Work out the finished part from the listing and answer in its coordinate system (mm). A direction names the side the tool comes from. Coordinates: 2 decimals unless noted, no trailing zeros. Write each loop counter-clockwise with the first axis right and the second up, starting at its lowest first coordinate (ties: lowest second). Pieces come first, ordered by that corner, then holes. Notation, with made-up numbers: (10.5, -23) -> (46.5, -23) arc R14 ccw to (46.5, 4) -> close; hole circle Ø1 at (87, 87.25). An arc over 180 degrees is marked (long way). Write each question's results on one line, items separated by ' | '. Start each with the question number.
Autodesk Inventor part; units mm, degrees
ref_plane "YZ Plane" through (0, 0, 0) normal (1, 0, 0) x (0, 1, 0)
ref_plane "XZ Plane" through (0, 0, 0) normal (0, 1, 0) x (-1, 0, 0)
ref_plane "XY Plane" through (0, 0, 0) normal (0, 0, 1) x (1, 0, 0)
sketch "Skizze1" plane through (0, 0, 0) normal (0, 0, 1) x (1, 0, 0)
  circle A0 centre (3.625, -20.7) radius 1.6
  circle A1 centre (3.625, -7) radius 1.6
  line L0 (7.8, -27.7) -> (7.8, -25.75)
  line L1 (7.8, -25.75) -> (7.25, -25.75)
  line L2 (7.25, -25.75) -> (7.25, 0)
  line L3 (0, 0) -> (7.25, 0)
  line L4 (0, -27.7) -> (0, 0)
  line L5 (0, -27.7) -> (7.8, -27.7)
  circle A2 centre (13.375, -20.7) radius 1.6
  circle A3 centre (13.375, -7) radius 1.6
  line L6 (9.2, -25.75) -> (9.2, -27.7)
  line L7 (9.2, -27.7) -> (17, -27.7)
  line L8 (17, 0) -> (17, -27.7)
  line L9 (9.75, 0) -> (17, 0)
  line L10 (9.75, 0) -> (9.75, -25.75)
  line L11 (9.75, -25.75) -> (9.2, -25.75)
  line L12 (0.5, 0) -> (17, 0)
  line L13 (17, 0) -> (17, -27.7)
  line L14 (17, -27.7) -> (0.5, -27.7)
  line L15 (0.5, -27.7) -> (0.5, 0)
  dimension "d0" = 0.5
extrude "Extrusion1" add sketch "Skizze1" along normal blind 5 contours A0 | A1 | L5 L15 L3 L2 L1 L0 | L0 L1 L2 L12 L10 L11 L6 L14 | L6 L11 L10 L9 L8 L7 | A2 | A3
sketch "Skizze2" plane through (0, 0, 5) normal (0, 0, 1) x (1, 0, 0)
  circle A0 centre (3.625, -7) radius 1.6
  circle A1 centre (13.375, -7) radius 1.6
  circle A2 centre (13.375, -20.7) radius 1.6
  circle A3 centre (3.625, -20.7) radius 1.6
  point P0 (0, 0)
extrude "Extrusion2" cut sketch "Skizze2" against normal blind 10
sketch "Skizze3" plane through (0, 0, 0) normal (0, 0, -1) x (-1, 0, 0)
  line L0 (-7.25, -25.75) -> (-7.25, 0)
  line L1 (-9.75, 0) -> (-9.75, -25.75)
  line L2 (-9.75, -25.75) -> (-7.25, -25.75)
  line L3 (-7.25, 0) -> (-9.75, 0)
  line L4 (-17, 0) -> (-0.5, 0)
  point P0 (0, 0)
  dimension "d5" = 2.5
extrude "Extrusion3" cut sketch "Skizze3" against normal blind 1.25
sketch "Skizze4" plane through (0, 0, 0) normal (0, 0, -1) x (-1, 0, 0)
  line L0 (-7.8, -27.7) -> (-7.8, -25.75)
  line L1 (-9.2, -25.75) -> (-9.2, -27.7)
  line L2 (-7.8, -27.7) -> (-9.2, -27.7)
  line L3 (-0.5, -27.7) -> (-17, -27.7)
  line L4 (-7.8, -25.75) -> (-9.2, -25.75)
  line L5 (-7.25, -25.75) -> (-9.75, -25.75)
  point P0 (0, 0)
  dimension "d8" = 1.4
extrude "Extrusion4" cut sketch "Skizze4" against normal blind 0.7
fillet "Rundung1" radius 2 2 edges at (17, 0, 2.5) (17, -27.7, 2.5)
sketch "Skizze5" plane through (0.5, 0, 5) normal (0, 1, 0) x (1, 0, 0)
  line L0 (0, 5) -> (7.3, 5)
  line L1 (8.7, 5) -> (14.5, 5)
  arc A0 (5.5, 5) -> (10.5, 5) centre (8, 5) ccw
  line L2 (8.7, 4.3) -> (7.3, 4.3)
  arc A1 (3, 5) -> (13, 5) centre (8, 5) ccw
  line L3 (13, 5) -> (10.5, 5)
  line L4 (5.5, 5) -> (3, 5)
  line L5 (14.5, 0) -> (0, 0)
  point P0 (-0.5, 5)
  point P1 (8, 4.3)
  dimension "d12" = 2.5
  dimension "d13" = 0
extrude "Extrusion5" add sketch "Skizze5" along normal blind 20
sketch "Skizze7" plane through (0, 0, 5) normal (0, 0, 1) x (1, 0, 0)
  circle A0 centre (3.625, -7) radius 3
  circle A1 centre (13.375, -7) radius 3
  circle A2 centre (13.375, -20.7) radius 1.6
  circle A3 centre (13.375, -20.7) radius 3
  circle A4 centre (3.625, -20.7) radius 3
  circle A5 centre (3.625, -7) radius 1.6
  circle A6 centre (13.375, -7) radius 1.6
  circle A7 centre (3.625, -20.7) radius 1.6
  point P0 (0, 0)
  dimension "d18" = 6
extrude "Extrusion7" cut sketch "Skizze7" against normal blind 2 contours A0 | A1 | A2 | A3 | A4 | A5 | A7
sketch "Skizze8" plane through (0.5, 20, 5) normal (0, 1, 0) x (1, 0, 0)
  point P0 (-0.5, 5)
sketch "Skizze9" plane through (0.5, 20, 5) normal (0, 1, 0) x (1, 0, 0)
  line L0 (13, 5) -> (10.5, 5)
  arc A0 (5.5, 5) -> (10.5, 5) centre (8, 5) ccw
  line L1 (5.5, 5) -> (3, 5)
  arc A1 (3, 5) -> (13, 5) centre (8, 5) ccw
  circle A2 centre (8, 5) radius 5
  line L2 (5.5, 5) -> (10.5, 5)
  point P0 (-0.5, 5)
  point P1 (3, 5)
  point P2 (13, 5)
extrude "Extrusion8" add sketch "Skizze9" along normal blind 2 contours A1 L1 A0 L0 | A0 L2
equation "\"d6\" = 0.5 * d5"
equation "\"d9\" = 0.5 * d8"
properties part number "NadelHalterLose"
1. Given pin 1 Ø1 at (x, z) = (2.5, 3.5) entering from +Y; pin 2 Ø5 at (x, y) = (3.625, -20.7) entering from -Z; pin 3 Ø1.5 at (x, y) = (4.5, -20.5) entering from +Z; pin 4 Ø0.7 at (x, y) = (8.5, -26.5) entering from -Z, each flat-ended and moving along its own axis, determine where each tip first touches the part or whether it passes through.
2. Find the intervals of material crossed by L1, parallel to Y at x = 3.5, z = 3.55; L2, parallel to Y at x = 4, z = 2.85; L3, parallel to Y at x = 8.75, z = 1.8, in increasing order.
3. Find section D-D on y = 16. Give the vertices of the cut face in (x, z), and give its area (3 significant figures).
4. Determine the mould class of faces 1 (the face through (8, 20, 1)), 2 (the face through (0.5, -14, 2)), 3 (the face through (16.43, -0.6, 2.54)), 4 (the face through (8, 0, 2)) for opening direction Y: pulls with the +Y half, pulls with the -Y half, needs draft (parallel to the pull), parting line crosses it, or undercut.
5. Find section C-C on y = -16. Give the vertices of the cut face in (x, z), and give its area (3 significant figures).
6. Find section B-B on z = 3.6. Give the vertices of the cut face in (x, y) (3 decimals), and give its area (3 significant figures).
7. For faces 5 (the face through (7.25, -13, 1)), 6 (the face through (8, 22, 2)), 7 (the face through (1.414, -4.972, 4.014)), 8 (the face through (3, 0, 3)), determine the directions among +Z, -Z, +X, -X, +Y, -Y from which every point of the face is accessible in a straight line to the end or side of a thin tool.
8. Find section A-A on y = -7. Give the vertices of the cut face in (x, z) (3 decimals), and give its area (3 significant figures).
Ans:
1) pin 1: stops at y = 0 | pin 2: stops at z = 0 | pin 3: stops at z = 3 | pin 4: stops at z = 0.7
2) L1: y = -27.7 to -23.7, -17.7 to -10, -4 to 0 | L2: y = -27.7 to -22.26, -19.14 to -8.56, -5.44 to 0 | L3: y = -27.7 to 0, 20 to 22
3) outline: (3.5, 0) -> (6, 0) arc R2.5 cw to (11, 0) -> (13.5, 0) arc R5 ccw to start | area: 29.5 mm²
4) face 1: undercut | face 2: needs draft | face 3: pulls with the +Y half | face 4: undercut
5) outline: (0.5, 0) -> (7.25, 0) -> (7.25, 1.25) -> (9.75, 1.25) -> (9.75, 0) -> (17, 0) -> (17, 5) -> (0.5, 5) -> close | area: 79.4 mm²
6) outline: (0.5, -27.7) -> (15, -27.7) arc R2 ccw to (17, -25.7) -> (17, -2) arc R2 ccw to (15, 0) -> (11.97, 0) -> (11.97, 22) -> (5.03, 22) -> (5.03, 0) -> (0.5, 0) -> close; hole circle Ø6 at (3.625, -20.7); hole circle Ø6 at (3.625, -7); hole circle Ø6 at (13.375, -20.7); hole circle Ø6 at (13.375, -7) | area: 495 mm²
7) face 5: -Z | face 6: +Z, -Z, +X, -X, +Y | face 7: +Z | face 8: +Z, -X, +Y
8) outline: (0.5, 0) -> (2.025, 0) -> (2.025, 3) -> (0.625, 3) -> (0.625, 5) -> (0.5, 5) -> close; (5.225, 0) -> (7.25, 0) -> (7.25, 1.25) -> (9.75, 1.25) -> (9.75, 0) -> (11.775, 0) -> (11.775, 3) -> (10.375, 3) -> (10.375, 5) -> (6.625, 5) -> (6.625, 3) -> (5.225, 3) -> close; (14.975, 0) -> (17, 0) -> (17, 5) -> (16.375, 5) -> (16.375, 3) -> (14.975, 3) -> close | area: 36.2 mm²
